Could you check a few things on this model? Use its own coordinates, in mm. A direction names the side the tool comes from. Coordinates: 2 decimals unless noted, no trailing zeros. Order: outer loops, then holes, each group sorted by start corner. A loop starts at its lowest first (then second) coordinate and runs counter-clockwise, first axis right, second up. Notation, with made-up numbers: (20.5, 45.5) -> (26.5, 45.5) arc R10 cw to (26.5, 62.5) -> close; hole circle Ø4 at (44.5, 53.5). An arc over 180 degrees is marked (long way). Use a Markdown table: item, result. Add a question column.
1) Which directions (+Z, -Z, +X, -X, +Y, -Y) give clear straight access to the entire face, cutting with the end or side of a thin tool? Please do faces 4 (the cylindrical face through (20.72, 4.51, 1.52)), 5 (the cylindrical face through (73, -24, 2)).
2) Will these pins go through, and if not, where does the flat tip stop? pin 1 Ø1.8 at (x, y) = (-95, 0) entering from -Z; pin 2 Ø0.9 at (x, z) = (-18, 1) entering from +Y.
3) If we section it at C-C (x = -40): Write out the boundary of the cut face in (y, z).
4) Thinking about a two-plate mould opening in X: for faces 1 (the flat face through (-19, -9, 3)), 2 (the flat face through (-10, 0, 2)), 3 (the cylindrical face through (-109, -23, 2)), which applies, +X half, -X half, draft (parallel to the pull), parting line (faces both ways), or undercut?
5) If we section it at A-A (z = 1.2): Write out the boundary of the cut face in (x, y).
6) If I drill on L1, parallel to Y at x = 60, z = 0.95; L2, parallel to Y at x = 8.5, z = 2.35; L3, parallel to X at y = 13, z = 1.85, over which ranges is the centre line in solid material (lowest first)? Write a range as [from, to].
7) If we section it at B-B (x = -12.5): Write out the boundary of the cut face in (y, z), plus the area to 3 significant figures.
```python
from build123d import *

# Parameters (mm, degrees)
SKETCH_1_W          = 185
SKETCH_1_H          = 40
EXTRUDE_1_DEPTH     = 3
SKETCH_2_R          = 1.5
CUT_EXTRUDE_1_DEPTH = 3
CUT_EXTRUDE_2_DEPTH = 3
FILLET_1_R          = 5
SKETCH_4_R          = 1.5
CUT_EXTRUDE_3_DEPTH = 3
CHAMFER_1_SIZE      = 0.5


with BuildPart() as part:
    # 草图1 → 凸台-拉伸1 (new body)
    with BuildSketch(Plane.XY):
        with Locations((-17.5, -5)):
            Rectangle(SKETCH_1_W, SKETCH_1_H)
    extrude(amount=EXTRUDE_1_DEPTH)

    # 草图2 → 切除-拉伸1 (cut)
    with BuildSketch(Plane.XY.offset(3)):
        with Locations((60, 0)):
            Circle(SKETCH_2_R)
        with Locations((-60, 0)):
            Circle(SKETCH_2_R)
    extrude(amount=-CUT_EXTRUDE_1_DEPTH, mode=Mode.SUBTRACT)

    # 草图3 → 切除-拉伸2 (cut)
    with BuildSketch(Plane.XY.offset(3)):
        with BuildLine():
            Line((-30, 30), (10, 30))
            ThreePointArc((10, 30), (25, 15), (10, 0))
            Line((10, 0), (-30, 0))
            ThreePointArc((-30, 0), (-45, 15), (-30, 30))
        make_face()
    extrude(amount=-CUT_EXTRUDE_2_DEPTH, mode=Mode.SUBTRACT)

    # 圆角1
    fillet_1_edges = [part.edges().sort_by_distance(p)[0] for p in [
        (75, -25, 1.5),
        (-110, -25, 1.5),
    ]]
    fillet(fillet_1_edges, radius=FILLET_1_R)

    # 草图4 → 切除-拉伸3 (cut)
    with BuildSketch(Plane.XY.offset(3)):
        with Locations((-95, 0)):
            Circle(SKETCH_4_R)
    extrude(amount=-CUT_EXTRUDE_3_DEPTH, mode=Mode.SUBTRACT)

    # 倒角1
    chamfer_1_edges = [part.edges().sort_by_distance(p)[0] for p in [
        (50, 15, 3),
        (-77.5, 15, 0),
        (-77.5, 15, 3),
        (50, 15, 0),
    ]]
    chamfer(chamfer_1_edges, length=CHAMFER_1_SIZE)


solid = part.part
```
Answer sheet:
| question | item | result |
|---|---|---|
| 1 | face 4 | +Z, -Z, +Y |
| 1 | face 5 | +Z, -Z, +X, -Y |
| 2 | pin 1 | through |
| 2 | pin 2 | y = 0 |
| 3 | outline | (-25, 0) -> (3.82, 0) -> (3.82, 3) -> (-25, 3) -> close |
| 4 | face 1 | draft |
| 4 | face 2 | undercut |
| 4 | face 3 | -X half |
| 5 | outline | (-110, -20) arc R5 ccw to (-105, -25) -> (70, -25) arc R5 ccw to (75, -20) -> (75, 15) -> (25, 15) arc R15 cw to (10, 0) -> (-30, 0) arc R15 cw to (-45, 15) -> (-110, 15) -> close; hole circle Ø3 at (-95, 0); hole circle Ø3 at (-60, 0); hole circle Ø3 at (60, 0) |
| 6 | L1 | [-25, -1.5], [1.5, 15] |
| 6 | L2 | [-25, 0] |
| 6 | L3 | [-110, -44.87], [24.87, 75] |
| 7 | outline | (-25, 0) -> (0, 0) -> (0, 3) -> (-25, 3) -> close |
| 7 | area | 75.0 mm2 |
